Job drawing, mm, ordinate dimensions from the low corner. One solid piece. Coordinates: 2 decimals unless noted, no trailing zeros. Order: outer loops, then holes, each group sorted by start corner. A loop starts at its lowest first (then second) coordinate and runs counter-clockwise, first axis right, second up. Notation, with made-up numbers: M 4,77.25 L 60,77.25 A26 ccw 60,92.25 Z; hole C 40,-0.75 d1. An arc over 180 degrees is marked long. Write item = value, one per line. Start each with the question number.
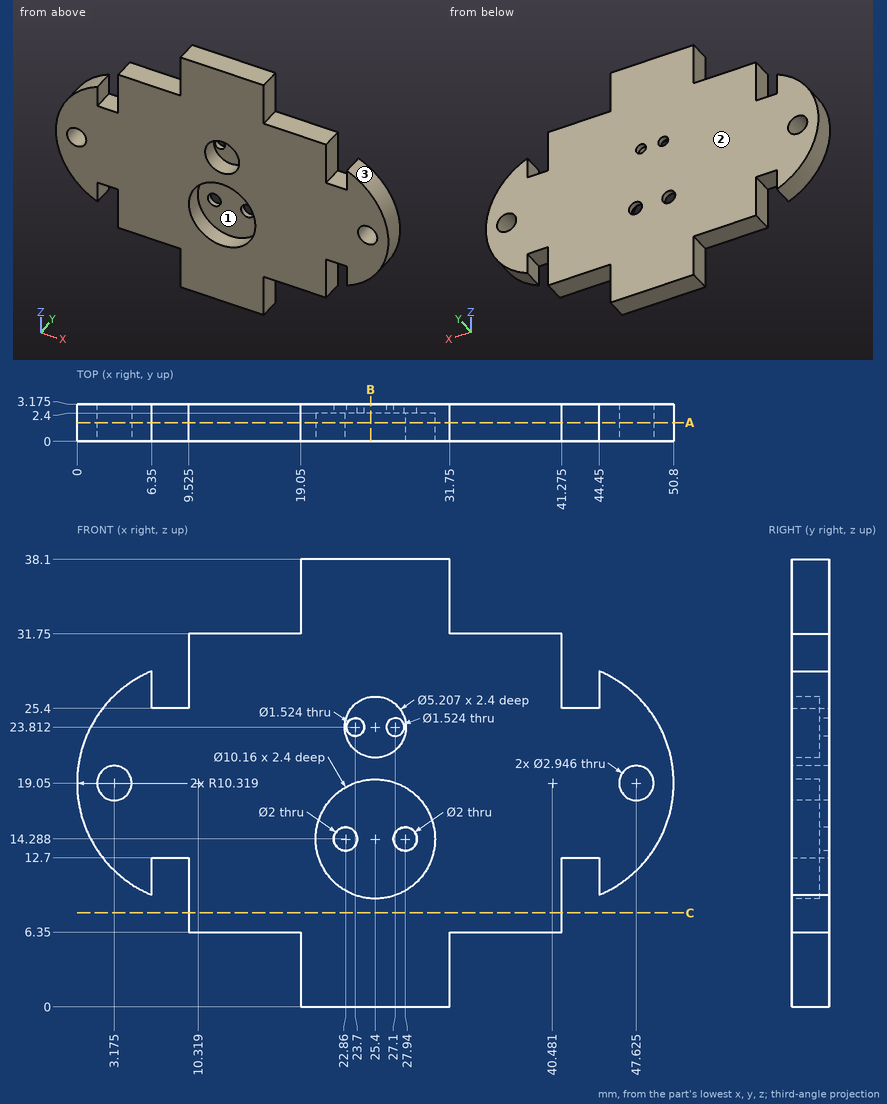
1. Flat gauge pins, fed straight in: pin 1 (5 mm diameter, centred on x = 26.5, z = 13, fed in from -Y); pin 2 (1 mm diameter, centred on y = 2, z = 9.5, fed in from +X); pin 3 (1 mm diameter, centred on x = 42.5, y = 2.5, fed in from -Z). Where does each tip first touch, or does it go through?
2. Slice it at C-C (z = 8). Write the cut outline in (x, y) (1 decimal), plus the area to 3 significant figures.
3. Probe L1, parallel to Z at x = 22.86, y = 2.75; L2, parallel to Z at x = 24, y = 2.2 (1 decimal); L3, parallel to Z at x = 33.5, y = 0.25. List the from-to ranges inside material, lowest first.
4. Slice it at B-B (x = 25). Write the cut outline in (y, z) (1 decimal).
5. Slice it at A-A (y = 1.6). Give the number of separate pieces and of enclosed holes in the cut face, plus the area to 3 significant figures.
6. Mould opens along Z. For the marked faces 1, 2 and 3 say: released by +Z, released by -Z, zero draft, split by the parting line, or undercut.
Calculated:
q1.pin_1 = 2.4
q1.pin_2 = 45.44
q1.pin_3 = 12.7
q2.outline = M 9.5,0 L 41.3,0 L 41.3,3.2 L 9.5,3.2 Z
q2.area = 101 mm²
q3.L1 = 0 to 13.29, 15.29 to 38.1
q3.L2 = 0 to 9.4, 19.2 to 21.6, 26 to 38.1
q3.L3 = 6.35 to 31.75
q4.outline = M 0,0 L 3.2,0 L 3.2,38.1 L 0,38.1 L 0,26.4 L 2.4,26.4 L 2.4,21.2 L 0,21.2 L 0,19.4 L 2.4,19.4 L 2.4,9.2 L 0,9.2 Z
q5.separate_pieces = 1
q5.enclosed_holes = 4
q5.area = 1,110 mm²
q6.face_1 = undercut
q6.face_2 = zero draft
q6.face_3 = split by the parting line
